CAD build for the part. Positions are in the model's coordinates, mm. Face numbers are marked on the shaded views. Coordinates: 2 decimals unless noted, no trailing zeros. Loops run counter-clockwise (first coordinate to the right, second up) from the corner with the lowest first, then second, coordinate; pieces in that order, holes last. Notation, with made-up numbers: (36.5, 3) -> (95.5, 3) arc R8 ccw to (95.5, 13) -> close; hole circle Ø9 at (6.5, 14.5). An arc over 180 degrees is marked (long way). Write each question's results on one line, items separated by ' | '.
from build123d import *

# Parameters (mm, degrees)
SKETCH1_W           = 16
SKETCH1_H           = 46
SKETCH1_R           = 2
BOSS_EXTRUDE1_DEPTH = 4
FILLET1_RADIUS      = 8
FILLET1_LENGTH      = 4
FILLET2_RADIUS      = 8
FILLET2_LENGTH      = 4


with BuildPart() as part:
    # Sketch1 → Boss-Extrude1 (new body)
    with BuildSketch(Plane(origin=(0, 0, 0), x_dir=(1, 0, 0), z_dir=(0, 1, 0))):
        Rectangle(SKETCH1_W, SKETCH1_H)
        with Locations(Location((0, -16, 0), (0, 0, 270))):
            Circle(SKETCH1_R, mode=Mode.SUBTRACT)
        with Locations(Location((0, 16, 0), (0, 0, 270))):
            Circle(SKETCH1_R, mode=Mode.SUBTRACT)
    extrude(amount=BOSS_EXTRUDE1_DEPTH)

    # Fillet1: full round fillet: the end face becomes a half cylinder, R = half its width
    fillet1_face = Plane((0, 2, 23), x_dir=(0, 1, 0), z_dir=(0, 0, 1))  # on the end face: x along it, z out of the body
    fillet1_slab = fillet1_face.offset(-FILLET1_RADIUS / 2) * Box(FILLET1_LENGTH, 2 * FILLET1_RADIUS, FILLET1_RADIUS, mode=Mode.PRIVATE)  # the body's end, R deep
    fillet1_round = Plane((0, 2, 15), x_dir=(0, 0, 1), z_dir=(0, 1, 0)) * Cylinder(FILLET1_RADIUS, FILLET1_LENGTH, mode=Mode.PRIVATE)  # its axis R under the face
    add(fillet1_slab - fillet1_round, mode=Mode.SUBTRACT)

    # Fillet2: full round fillet: the end face becomes a half cylinder, R = half its width
    fillet2_face = Plane((0, 2, -23), x_dir=(0, 1, 0), z_dir=(0, 0, -1))  # on the end face: x along it, z out of the body
    fillet2_slab = fillet2_face.offset(-FILLET2_RADIUS / 2) * Box(FILLET2_LENGTH, 2 * FILLET2_RADIUS, FILLET2_RADIUS, mode=Mode.PRIVATE)  # the body's end, R deep
    fillet2_round = Plane((0, 2, -15), x_dir=(0, 0, -1), z_dir=(0, 1, 0)) * Cylinder(FILLET2_RADIUS, FILLET2_LENGTH, mode=Mode.PRIVATE)  # its axis R under the face
    add(fillet2_slab - fillet2_round, mode=Mode.SUBTRACT)


solid = part.part
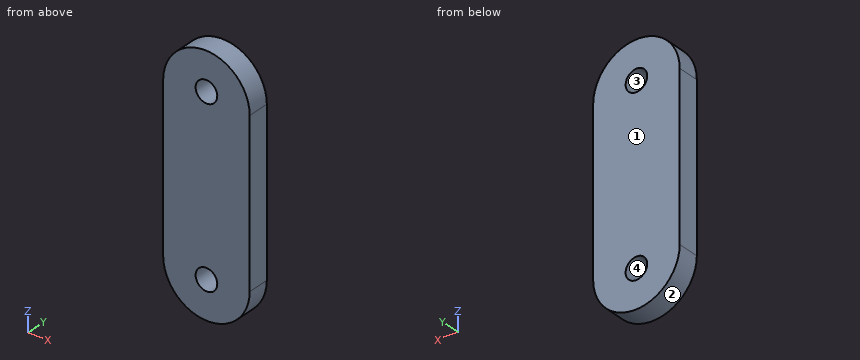
1) Slice it at A-A (y = 3.35). Write the cut outline in (x, z).
Outcome:
outline: (-8, -15) arc R8 ccw to (8, -15) -> (8, 15) arc R8 ccw to (-8, 15) -> close; hole circle Ø4 at (0, -16); hole circle Ø4 at (0, 16)
2) Drill centre lines: L1, parallel to Z at x = -1.25, y = 1.3; L2, parallel to X at y = 1.5, z = -16; L3, parallel to Z at x = -6.5, y = 3.05. Where is each one in solid material? Low to high. Write a range as from..to.
Outcome:
L1: z = -22.9..-17.56, -14.44..14.44, 17.56..22.9 | L2: x = -7.94..-2, 2..7.94 | L3: z = -19.66..19.66
3) Slice it at B-B (z = 16). Write the cut outline in (x, y), then the cut area to 3 significant figures.
Outcome:
outline: (-7.94, 0) -> (-2, 0) -> (-2, 4) -> (-7.94, 4) -> close; (2, 0) -> (7.94, 0) -> (7.94, 4) -> (2, 4) -> close | area: 47.5 mm^2
4) Slice it at D-D (z = -19.5). Write the cut outline in (x, y).
Outcome:
outline: (-6.61, 0) -> (6.61, 0) -> (6.61, 4) -> (-6.61, 4) -> close
5) Two-plate mould, pull along X, no slides. Class the marked faces 1, 2, 3 and 4: pulls with the +X half, pulls with the -X half, needs draft (parallel to the pull), parting line crosses it, or undercut.
Outcome:
face 1: needs draft | face 2: parting line crosses it | face 3: undercut | face 4: undercut
6) Slice it at C-C (x = -5.25). Write the cut outline in (y, z), then the cut area to 3 significant figures.
Outcome:
outline: (0, -21.04) -> (4, -21.04) -> (4, 21.04) -> (0, 21.04) -> close | area: 168 mm^2
